from build123d import *

# Parameters (mm, degrees)
SKETCH1_W           = 100
SKETCH1_H           = 100
BOSS_EXTRUDE2_DEPTH = 3.18
SKETCH2_R           = 1.55
SKETCH2_W           = 3.18
SKETCH2_H           = 40.125
CUT_EXTRUDE1_DEPTH  = 4.18


with BuildPart() as part:
    # Sketch1 → Boss-Extrude2 (new body)
    with BuildSketch(Plane.XY):
        Rectangle(SKETCH1_W, SKETCH1_H)
    extrude(amount=BOSS_EXTRUDE2_DEPTH)

    # Sketch2 → Cut-Extrude1 (cut, through all)
    with BuildSketch(Plane.XY.offset(3.18)):
        with Locations((-48, 0)):
            Circle(SKETCH2_R)
        Polygon((-10, 50), (-10, 46.82), (-1.5, 46.82), (-1.5, 42.82), (-3.25, 42.82), (-3.25, 39.82), (-1.5, 39.82), (-1.5, 37), (1.5, 37), (1.5, 39.82), (3.25, 39.82), (3.25, 42.82), (1.5, 42.82), (1.5, 46.82), (10, 46.82), (10, 50), align=None)
        with Locations((-48.41, 29.9375)):
            Rectangle(SKETCH2_W, SKETCH2_H)
        with Locations((-48.41, -29.9375)):
            Rectangle(SKETCH2_W, SKETCH2_H)
    cut_extrude1 = extrude(amount=-CUT_EXTRUDE1_DEPTH, mode=Mode.SUBTRACT)

    # Mirror1: Cut-Extrude1 across plane
    add(cut_extrude1.mirror(Plane.ZX), mode=Mode.SUBTRACT)

    # Mirror3: Cut-Extrude1 across plane
    add(cut_extrude1.mirror(Plane(origin=(0, 0, 0), x_dir=(0, 0, 1), z_dir=(1, 0, 0))), mode=Mode.SUBTRACT)


solid = part.part
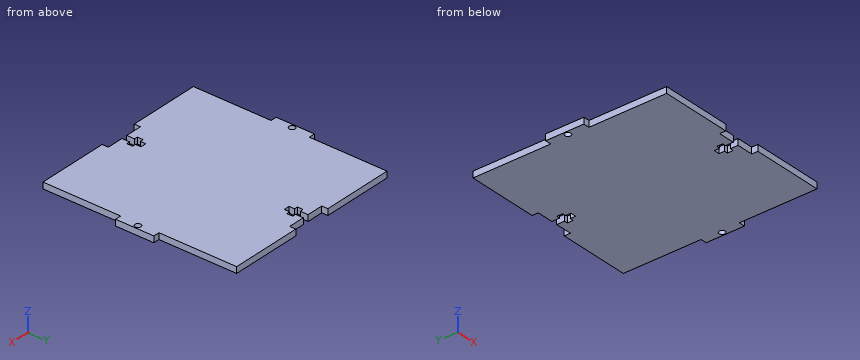
Design review of the part built by this model. Coordinates are the model's own, in mm. Give positions to 0.01 mm unless a question says otherwise; leave off trailing zeros. Loops run counter-clockwise (first coordinate to the right, second up) from the corner with the lowest first, then second, coordinate; pieces in that order, holes last. Notation, with made-up numbers: M -7,53.25 L 30,53.25 A18 ccw 30,68.25 Z; hole C 63.25,4 d5. An arc over 180 degrees is marked long. Write item = value, one per line.
Q1. We need section C-C (y = 0). Give the boundary of the cut face in (x, z), plus the area to 3 significant figures.
Output values:
outline = M -50,0 L -49.55,0 L -49.55,3.18 L -50,3.18 Z; M -46.45,0 L 46.45,0 L 46.45,3.18 L -46.45,3.18 Z; M 49.55,0 L 50,0 L 50,3.18 L 49.55,3.18 Z
area = 298 mm^2
Q2. We need section A-A (y = -41). Give the boundary of the cut face in (x, z).
Output values:
outline = M -46.82,0 L -3.25,0 L -3.25,3.18 L -46.82,3.18 Z; M 3.25,0 L 46.82,0 L 46.82,3.18 L 3.25,3.18 Z
Q3. We need section B-B (x = -48). Give the boundary of the cut face in (y, z) (3 decimals).
Output values:
outline = M -9.875,0 L -1.55,0 L -1.55,3.18 L -9.875,3.18 Z; M 1.55,0 L 9.875,0 L 9.875,3.18 L 1.55,3.18 Z
Q4. We need section D-D (z = 2.7). Count the separate pieces of the cut face and the enclosed holes in it, plus the area to 3 significant figures.
Output values:
separate_pieces = 1
enclosed_holes = 2
area = 9,270 mm^2
Q5. Insertion check: pin 1 (1.5 mm diameter, centred on y = -41.5, z = 2, fed in from +X); pin 2 (1.5 mm diameter, centred on y = -41.5, z = 1, fed in from -X); pin 3 (0.9 mm diameter, centred on x = 0.5, z = 2, fed in from -Y). Each pin has a flat end and moves straight along its axis. Give the tip position at first contact, or say it passes through.
Output values:
pin_1 = 46.82
pin_2 = -46.82
pin_3 = -37
Q6. To check wall thickness, follow line 1 (Y direction, x = -48, z = 1.7) (3 decimals); line 2 (X direction, y = 27, z = 1.8); line 3 (X direction, y = -1, z = 2.1). State the ranges of each line that lie inside material, in increasing order. Write a range as [from, to].
Output values:
line_1 = [-9.875, -1.55], [1.55, 9.875]
line_2 = [-46.82, 46.82]
line_3 = [-50, -49.18], [-46.82, 46.82], [49.18, 50]
